The figure shows three views and two pictorial views of one solid part (mm, origin at its lowest corner). Answer the questions. Coordinates: 2 decimals unless noted, no trailing zeros. Loops run counter-clockwise (first coordinate to the right, second up) from the corner with the lowest first, then second, coordinate; pieces in that order, holes last. Notation, with made-up numbers: M 24,-25 L 73,-25 A17 ccw 73,6 Z; hole C 15,0.25 d9. An arc over 180 degrees is marked long. Answer as a JSON object with one key per item and string values. Group by question number.
1. A cutting plane is placed at A-A on x = 1.75. Give the vertices of the cut face in (y, z) (1 decimal), and give its area (3 significant figures).
2. A cutting plane is placed at B-B on y = 17.25. Give the vertices of the cut face in (x, z) (1 decimal).
3. Straight lines are drawn through the part: L1, parallel to Y at x = 5, z = 3.3 (3 decimals); L2, parallel to Z at x = 6, y = 18. For each, find the intervals that lie inside material, in ascending order.
4. A cutting plane is placed at C-C on z = 2.1. Give the vertices of the cut face in (x, y) (3 decimals), and give its area (3 significant figures).
5. Determine the mould class of the marked faces 1, 2 and 3 for opening direction Z: released by +Z, released by -Z, zero draft, split by the parting line, or undercut.
6. Given pin 1 (1.1 mm diameter, centred on x = 9, z = 3, fed in from +Y) (3 decimals), flat-ended and moving along its own axis, determine where the tip first touches the part or whether it passes through.
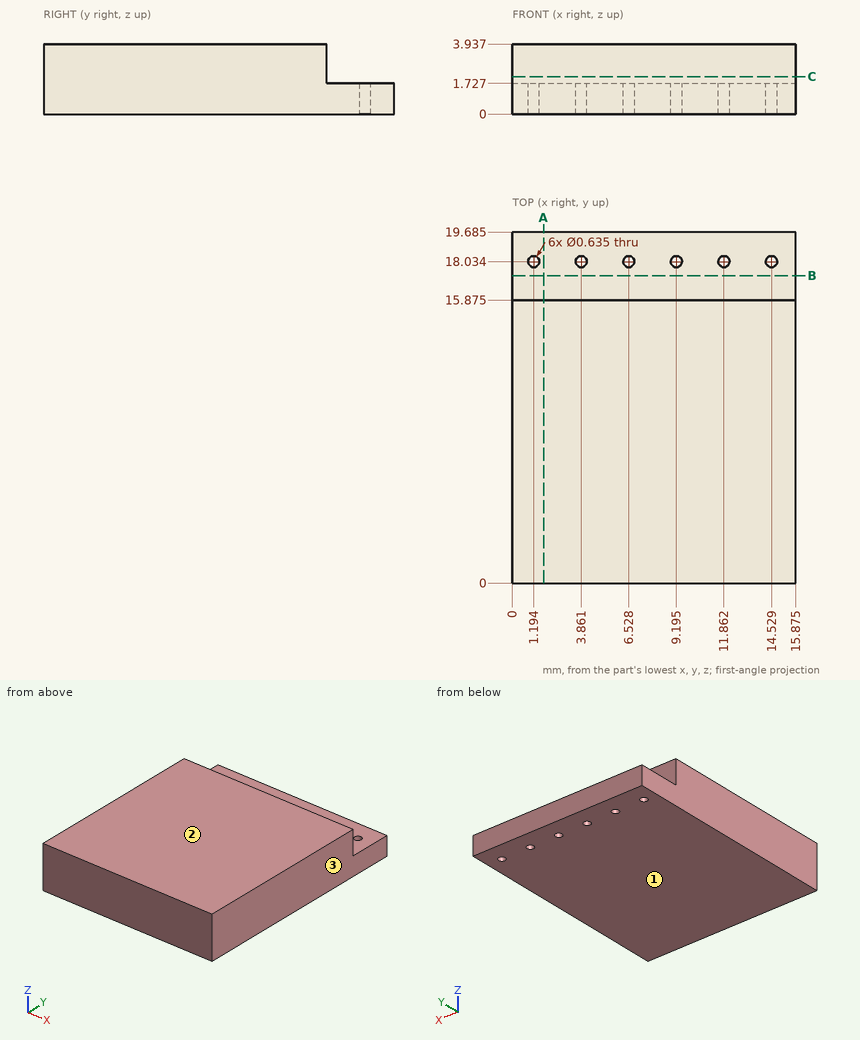
From the geometry:
{
 "1": {"outline": "M 0,0 L 19.7,0 L 19.7,1.7 L 15.9,1.7 L 15.9,3.9 L 0,3.9 Z", "area": "69.1 mm²"},
 "2": {"outline": "M 0,0 L 15.9,0 L 15.9,1.7 L 0,1.7 Z"},
 "3": {"L1": "y = 0 to 15.875", "L2": "z = 0 to 1.73"},
 "4": {"outline": "M 0,0 L 15.875,0 L 15.875,15.875 L 0,15.875 Z", "area": "252 mm²"},
 "5": {"face 1": "released by -Z", "face 2": "released by +Z", "face 3": "zero draft"},
 "6": {"pin 1": "stops at y = 15.875"}
}
